Check sheet for the drawn part. Datum: minimum x, y, z corner. Units: mm. A direction names the side the tool comes from. Give positions to 0.01 mm unless a question says otherwise; leave off trailing zeros. Order: outer loops, then holes, each group sorted by start corner. A loop starts at its lowest first (then second) coordinate and runs counter-clockwise, first axis right, second up. Notation, with made-up numbers: M 66,32.25 L 97,32.25 A13 cw 97,42.25 Z; hole C 3,24.25 d8. An arc over 180 degrees is marked long. Answer as CSV lines item,"result". Start each with the question number.
Q1. Section check A-A, the plane y = 22.5. Record the boundary of the cut face in (x, z).
Q2. Set-up check for the marked faces 1, 2 and 3: record each of +Z, -Z, +X, -X, +Y, -Y from which the full face is reachable in a straight line by a thin tool's end or side.
Q3. Section check D-D, the plane x = 43. Record the boundary of the cut face in (y, z).
Q4. Section check B-B, the plane z = 85. Record the boundary of the cut face in (x, y).
Q5. Go/stop test with flat-tipped pins: pin 1 (5 mm diameter, centred on x = 83.5, y = 17.5, fed in from -Z); pin 2 (1.5 mm diameter, centred on x = 28, y = 30.5, fed in from +Z); pin 3 (13 mm diameter, centred on y = 22.5, z = 85, fed in from -X). Record where each tip stops, or that it passes through.
Q6. Thickness scan on line 1 (Y direction, x = 15, z = 1.3); line 2 (Z direction, x = 79, y = 35); line 3 (Z direction, x = 23, y = 29). Record the ranges inside material, lowest first.
Q7. Section check C-C, the plane y = 11. Record the boundary of the cut face in (x, z).
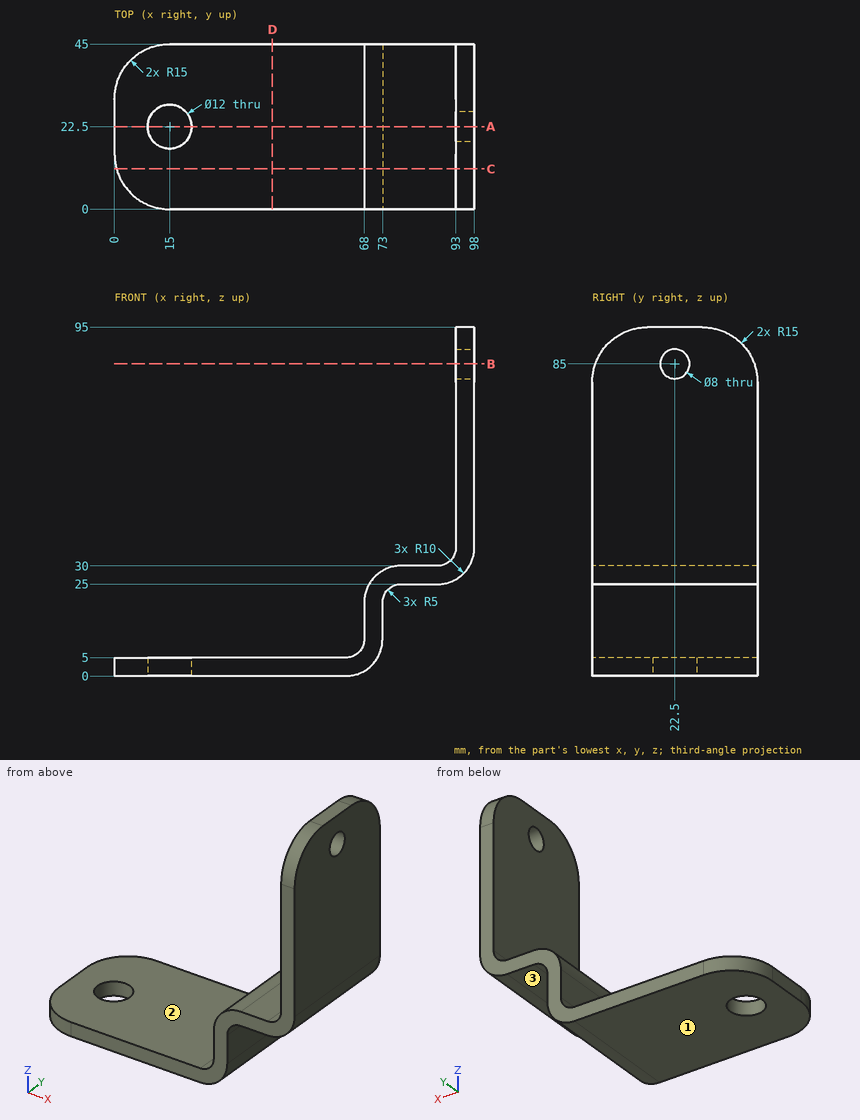
Answer block:
1,outline,"M 0,0 L 9,0 L 9,5 L 0,5 Z; M 21,0 L 63,0 A10 ccw 73,10 L 73,20 A5 cw 78,25 L 88,25 A10 ccw 98,35 L 98,81 L 93,81 L 93,35 A5 cw 88,30 L 78,30 A10 ccw 68,20 L 68,10 A5 cw 63,5 L 21,5 Z; M 93,89 L 98,89 L 98,95 L 93,95 Z"
2,face 1,"-Z, +X, -X, +Y, -Y"
2,face 2,"+Z, -X, +Y, -Y"
2,face 3,"-Z, +X, +Y, -Y"
3,outline,"M 0,0 L 45,0 L 45,5 L 0,5 Z"
4,outline,"M 93,0.86 L 98,0.86 L 98,18.5 L 93,18.5 Z; M 93,26.5 L 98,26.5 L 98,44.14 L 93,44.14 Z"
5,pin 1,"stops at z = 25"
5,pin 2,"stops at z = 5"
5,pin 3,"stops at x = 93"
6,line 1,"y = 0 to 16.5, 28.5 to 45"
6,line 2,"z = 25 to 30"
6,line 3,"z = 0 to 5"
7,outline,"M 0.54,0 L 63,0 A10 ccw 73,10 L 73,20 A5 cw 78,25 L 88,25 A10 ccw 98,35 L 98,94.46 L 93,94.46 L 93,35 A5 cw 88,30 L 78,30 A10 ccw 68,20 L 68,10 A5 cw 63,5 L 0.54,5 Z"
